Job drawing, mm, ordinate dimensions from the low corner. One solid piece. A direction names the side the tool comes from. Round coordinates to 2 decimals unless told otherwise and drop trailing zeros. Loops run counter-clockwise (first coordinate to the right, second up) from the corner with the lowest first, then second, coordinate; pieces in that order, holes last. Notation, with made-up numbers: M -24,87.25 L -7,87.25 A22 ccw -7,124.25 Z; hole C 79.5,8.25 d5. An arc over 180 degrees is marked long. Write each question's results on one line, items separated by ' | '. Start each with the question number.
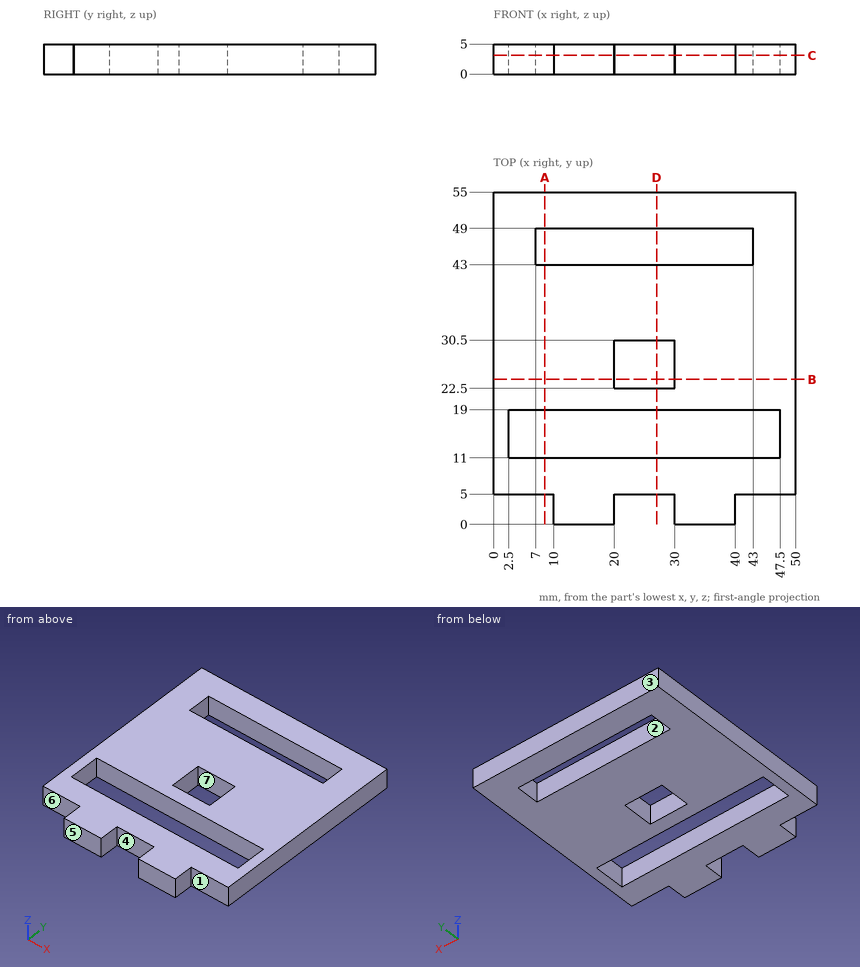
Item 1: Drop flat-ended pins along their axis: pin 1 (2.5 mm diameter, centred on x = 26, z = 2.5, fed in from -Y); pin 2 (1.5 mm diameter, centred on y = 3.5, z = 2, fed in from +X). Give the stop position or say it passes through.
Item 2: Drill centre lines: line 1 along Y through (x, z) = (39.5, 4.65); line 2 along X through (y, z) = (30, 3); line 3 along Y through (x, z) = (47, 1.45). Where is each one in solid material? Low to high. Write a range as [from, to].
Item 3: Saw through at C-C, the plane z = 3.1. Give the cut face in (x, y), then the cut area to 3 significant figures.
Item 4: Saw through at B-B, the plane y = 24. Give the cut face in (x, z).
Item 5: Saw through at D-D, the plane x = 27. Give the cut face in (y, z), then the cut area to 3 significant figures.
Item 6: Saw through at A-A, the plane x = 8.5. Give the cut face in (y, z).
Item 7: Tool access for the marked faces 1, 2, 3, 4 and 5: list every direction of +Z, -Z, +X, -X, +Y, -Y with a clear straight run to the whole face (end or side of a thin tool).
Item 8: Mould opens along X. For the marked faces 6 and 7 say: released by +X, released by -X, zero draft, split by the parting line, or undercut.
Working result:
1) pin 1: stops at y = 5 | pin 2: stops at x = 40
2) line 1: y = [0, 11], [19, 43], [49, 55] | line 2: x = [0, 20], [30, 50] | line 3: y = [5, 11], [19, 55]
3) outline: M 0,5 L 10,5 L 10,0 L 20,0 L 20,5 L 30,5 L 30,0 L 40,0 L 40,5 L 50,5 L 50,55 L 0,55 Z; hole M 2.5,11 L 47.5,11 L 47.5,19 L 2.5,19 Z; hole M 7,43 L 43,43 L 43,49 L 7,49 Z; hole M 20,22.5 L 30,22.5 L 30,30.5 L 20,30.5 Z | area: 1,940 mm²
4) outline: M 0,0 L 20,0 L 20,5 L 0,5 Z; M 30,0 L 50,0 L 50,5 L 30,5 Z
5) outline: M 5,0 L 11,0 L 11,5 L 5,5 Z; M 19,0 L 22.5,0 L 22.5,5 L 19,5 Z; M 30.5,0 L 43,0 L 43,5 L 30.5,5 Z; M 49,0 L 55,0 L 55,5 L 49,5 Z | area: 140 mm²
6) outline: M 5,0 L 11,0 L 11,5 L 5,5 Z; M 19,0 L 43,0 L 43,5 L 19,5 Z; M 49,0 L 55,0 L 55,5 L 49,5 Z
7) face 1: +Z, -Z, +X, -Y | face 2: +Z, -Z | face 3: +Z, -Z, +X, -X, +Y | face 4: +Z, -Z, -Y | face 5: +Z, -Z, +X, -X, -Y
8) face 6: zero draft | face 7: undercut
